For this review, take the finished solid that the model builds, in its own axes (mm). Face numbers are marked on the shaded views. A direction names the side the tool comes from. Give positions to 0.01 mm unless a question says otherwise; leave off trailing zeros. Write each loop counter-clockwise with the first axis right and the second up, starting at its lowest first coordinate (ties: lowest second). Pieces come first, ordered by that corner, then holes. Notation, with made-up numbers: (61, -9.75) -> (72, -9.75) arc R31 ccw to (72, 23.25) -> close; hole circle Ø8 at (51.25, -37). An arc over 180 degrees is marked (long way). Write item = value, one per line.
```python
from build123d import *

# Parameters (mm, degrees)
SKETCH2_R           = 1.5
BOSS_EXTRUDE1_DEPTH = 6
CUT_EXTRUDE1_DEPTH  = 1


with BuildPart() as part:
    # Sketch1 → Revolve1 (revolve)
    with BuildSketch(Plane(origin=(0, 0, 0), x_dir=(0, 0, -1), z_dir=(1, 0, 0))):
        with BuildLine():
            Line((0, 0), (0, 1.65))
            Line((0, 1.65), (-1, 1.65))
            ThreePointArc((-1, 1.65), (-2.075469546, 1.016421323), (-2.8, 0))
            Line((-2.8, 0), (0, 0))
        make_face()
    revolve(axis=Axis((0, 4.725289413, 0), (0, -1, 0)))

    # Sketch2 → Boss-Extrude1 (add)
    with BuildSketch(Plane.XZ):
        Circle(SKETCH2_R)
    extrude(amount=BOSS_EXTRUDE1_DEPTH)

    # Sketch3 → Cut-Extrude1 (cut)
    with BuildSketch(Plane(origin=(0, 1.65, 0), x_dir=(1, 0, 0), z_dir=(0, 1, 0))):
        Polygon((0, 1), (-0.866025404, 0.5), (-0.866025404, -0.5), (0, -1), (0.866025404, -0.5), (0.866025404, 0.5), align=None)
    extrude(amount=-CUT_EXTRUDE1_DEPTH, mode=Mode.SUBTRACT)


solid = part.part
```
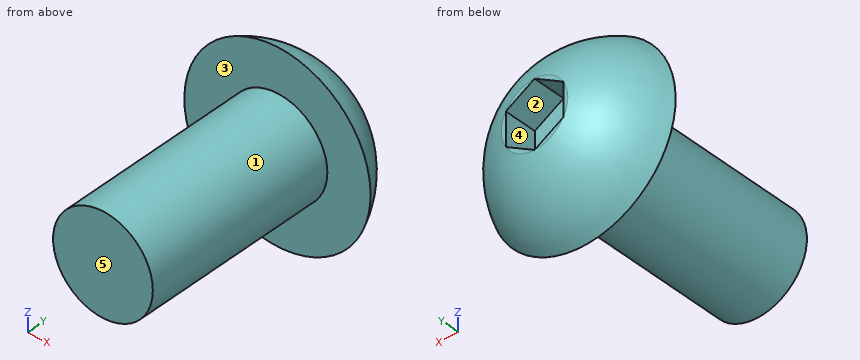
(1) The part is to be moulded in two halves that separate along Z. For the marked faces 1, 2 and 3, say which applies: released by +Z, released by -Z, zero draft, split by the parting line, or undercut.
Answers below:
face_1 = split by the parting line
face_2 = undercut
face_3 = zero draft
(2) For pin 1 (1 mm diameter, centred on x = -2, y = 0, fed in from +Z); pin 2 (2 mm diameter, centred on x = -1, y = 0.5, fed in from +Z); pin 3 (1.5 mm diameter, centred on y = -3.5, z = -0.5, fed in from -X), all flat-tipped, find the tip position at first contact; note any pin that passes through.
Answers below:
pin_1 = 2.36
pin_2 = 2.8
pin_3 = -1.5
(3) Tool access review of the marked faces 4 and 5: name each direction out of +Z, -Z, +X, -X, +Y, -Y from which nothing blocks a thin tool from reaching the whole face with its end or side.
Answers below:
face_4 = +Y
face_5 = +Z, -Z, +X, -X, -Y
(4) To check wall thickness, follow probe 1 along X at (y, z) = (-0.25, -0.05); probe 2 along Z at (x, y) = (-0.2, 1.25); probe 3 along X at (y, z) = (-0.75, -0.4). State the ranges of each line that lie inside material, in increasing order.
Answers below:
probe_1 = -1.5 to 1.5
probe_2 = -1.78 to -0.88, 0.88 to 1.78
probe_3 = -1.45 to 1.45
(5) Take a section at A-A (y = -2.75). Write out the cut boundary in (x, z).
Answers below:
outline = circle Ø3 at (0, 0)
